Verification items for the finished model (mm, model axes). A direction names the side the tool comes from. Round coordinates to 2 decimals unless told otherwise and drop trailing zeros. Write each loop counter-clockwise with the first axis right and the second up, starting at its lowest first coordinate (ties: lowest second). Pieces come first, ordered by that corner, then holes. Notation, with made-up numbers: M 5.25,47 L 30.25,47 A30 ccw 30.25,79 Z; hole C 29,66.5 d4. An arc over 180 degrees is marked long. One line per item, written item: value. Start each with the question number.
Item 1: Thickness scan on probe 1 along X at (y, z) = (1.95, 0); probe 2 along X at (y, z) = (3.4, -5.5); probe 3 along Z at (x, y) = (-40.5, 2.8). Record the ranges inside material, lowest first. Write a range as from..to.
Item 2: Tool access check on faces 1 (the face through (-29, 2, 0)), 2 (the face through (-1, 0, 0)). Record the directions out of +Z, -Z, +X, -X, +Y, -Y that give a thin tool (end or side, any length) a straight path to the whole face; none if there is none.
Item 3: Section check D-D, the plane x = 35.5. Record the cut outline in (y, z), then the cut area to 3 significant figures.
Item 4: Section check B-B, the plane z = 0. Record the cut outline in (x, y), then the cut area to 4 significant figures.
Item 5: Gauge pin test, flat end, axial feed: pin 1 (20 mm diameter, centred on x = 35.5, z = 0, fed in from -Y). Record the tip position at first contact, or that the pin passes through.
Item 6: Draft check along X on faces 3 (the face through (-1, 2, 28)), 4 (the face through (-38, 2, 7)), 5 (the face through (-90, 2, 0)), 6 (the face through (-46.5, 2, 0)). Enter one of: +X half, -X half, draft (parallel to the pull), parting line (faces both ways), or undercut.
Item 7: Section check C-C, the plane x = -41. Record the cut outline in (y, z), then the cut area to 3 significant figures.
Item 8: Section check A-A, the plane y = 2.2. Record the cut outline in (x, z).
from build123d import *

# Parameters (mm, degrees)
IZIM1_W                     = 180
IZIM1_H                     = 56
IZIM1_R                     = 11
IZIM1_W_2                   = 17.5
IZIM1_H_2                   = 14
Y_KSEKLIK_EKSTR_ZYON1_DEPTH = 5


with BuildPart() as part:
    # Çizim1 → Yükseklik-Ekstrüzyon1 (new body)
    with BuildSketch(Plane(origin=(0, 0, 0), x_dir=(1, 0, 0), z_dir=(0, 1, 0))):
        Rectangle(IZIM1_W, IZIM1_H)
        with Locations(Location((35.5, 0, 0), (0, 0, 270))):
            Circle(IZIM1_R, mode=Mode.SUBTRACT)
        with Locations((-37.75, 0)):
            Rectangle(IZIM1_W_2, IZIM1_H_2, mode=Mode.SUBTRACT)
    extrude(amount=Y_KSEKLIK_EKSTR_ZYON1_DEPTH)


solid = part.part
Response values:
1. probe 1: x = -90..-46.5, -29..24.5, 46.5..90
1. probe 2: x = -90..-46.5, -29..25.97, 45.03..90
1. probe 3: z = -28..-7, 7..28
2. face 1: +Y, -Y
2. face 2: +Z, -Z, +X, -X, -Y
3. outline: M 0,-28 L 5,-28 L 5,-11 L 0,-11 Z; M 0,11 L 5,11 L 5,28 L 0,28 Z
3. area: 170 mm2
4. outline: M -90,0 L -46.5,0 L -46.5,5 L -90,5 Z; M -29,0 L 24.5,0 L 24.5,5 L -29,5 Z; M 46.5,0 L 90,0 L 90,5 L 46.5,5 Z
4. area: 702.5 mm2
5. pin 1: passes through
6. face 3: draft
6. face 4: undercut
6. face 5: -X half
6. face 6: undercut
7. outline: M 0,-28 L 5,-28 L 5,-7 L 0,-7 Z; M 0,7 L 5,7 L 5,28 L 0,28 Z
7. area: 210 mm2
8. outline: M -90,-28 L 90,-28 L 90,28 L -90,28 Z; hole M -46.5,-7 L -29,-7 L -29,7 L -46.5,7 Z; hole C 35.5,0 d22
